```python
from build123d import *

# Parameters (mm, degrees)
SKETCH_1_W             = 67
SKETCH_1_H             = 62
EXTRUDE_1_DEPTH        = 10
SKETCH_3_W             = 14
SKETCH_3_H             = 20
EXTRUDE_2_DEPTH        = 12.5
SKETCH_4_W             = 10
SKETCH_4_H             = 65
EXTRUDE_3_DEPTH        = 67
SKETCH_5_W             = 67
SKETCH_5_H             = 44
EXTRUDE_4_DEPTH        = 8
EXTRUDE_5_DEPTH        = 20
CUT_EXTRUDE_START      = -6
CUT_EXTRUDE_1_DEPTH    = 8
EXTRUDE_6_DEPTH        = 6
SKETCH_9_R             = 3
CUT_EXTRUDE_2_DEPTH    = 23
SKETCH_10_W            = 24
SKETCH_10_H            = 23.8
EXTRUDE_7_DEPTH        = 8
SKETCH_12_W            = 14
SKETCH_12_H            = 20
EXTRUDE_8_DEPTH        = 11.5
SKETCH_13_R            = 0.95
CUT_EXTRUDE_4_DEPTH    = 8
SKETCH_14_W            = 8
SKETCH_14_H            = 6
EXTRUDE_9_DEPTH        = 11.8
SKETCH_15_R            = 0.95
CUT_EXTRUDE_5_DEPTH    = 11.8
SKETCH_16_W            = 3
SKETCH_16_H            = 6
EXTRUDE_10_DEPTH       = 12
FILLET_1_RADIUS        = 3
FILLET_1_LENGTH        = 3
SKETCH_17_R            = 1.75
CUT_EXTRUDE_6_DEPTH    = 7
SKETCH_18_R            = 3
EXTRUDE_11_DEPTH       = 36.5
FILLET_2_R             = 3
FILLET_2_OF_MIRROR_1_R = 3
SKETCH_20_R            = 1.75
CUT_EXTRUDE_7_DEPTH    = 35
SKETCH_21_W            = 15
SKETCH_21_H            = 55
CUT_EXTRUDE_8_DEPTH    = 35
SKETCH_24_R            = 1.75
CUT_EXTRUDE_11_DEPTH   = 18
SKETCH_25_R            = 1.5
CUT_EXTRUDE_12_DEPTH   = 10
FILLET_3_R             = 4
SKETCH_26_W            = 10.3
SKETCH_26_H            = 3.8
EXTRUDE_12_DEPTH       = 1
SKETCH_27_R            = 1.4
CUT_EXTRUDE_13_DEPTH   = 4


with BuildPart() as part:
    # 草图1 → 凸台-拉伸1 (new body)
    with BuildSketch(Plane(origin=(0, 0, 0), x_dir=(1, 0, 0), z_dir=(0, 1, 0))):
        Rectangle(SKETCH_1_W, SKETCH_1_H)
    extrude(amount=EXTRUDE_1_DEPTH)

    # 草图3 → 凸台-拉伸2 (add)
    with BuildSketch(Plane(origin=(0, 10, 0), x_dir=(1, 0, 0), z_dir=(0, 1, 0))):
        with Locations((-26.5, 26)):
            Rectangle(SKETCH_3_W, SKETCH_3_H)
    extrude(amount=EXTRUDE_2_DEPTH)

    # 草图4 → 凸台-拉伸3 (add)
    with BuildSketch(Plane.ZY.offset(33.5)):
        with Locations((-11, 42.5)):
            Rectangle(SKETCH_4_W, SKETCH_4_H)
    extrude(amount=-EXTRUDE_3_DEPTH)

    # 草图5 → 凸台-拉伸4 (add)
    with BuildSketch(Plane(origin=(0, 75, 0), x_dir=(1, 0, 0), z_dir=(0, 1, 0))):
        with Locations((0, -6)):
            Rectangle(SKETCH_5_W, SKETCH_5_H)
    extrude(amount=-EXTRUDE_4_DEPTH)

    # 草图6 → 凸台-拉伸5 (add)
    with BuildSketch(Plane(origin=(33.5, 0, 0), x_dir=(0, 0, -1), z_dir=(1, 0, 0))):
        with BuildLine():
            Line((-28, 60), (-28, 67))
            Line((-28, 67), (-8, 67))
            Line((-8, 67), (-8, 60))
            ThreePointArc((-8, 60), (-18, 50), (-28, 60))
        make_face()
    extrude_5 = extrude(amount=-EXTRUDE_5_DEPTH)

    # 草图7 → 切除-拉伸1 (cut)
    with BuildSketch(Plane(origin=(33.5, 0, 0), x_dir=(0, 0, -1), z_dir=(1, 0, 0)).offset(CUT_EXTRUDE_START)):
        with BuildLine():
            Line((-28, 60), (-28, 70.000230089))
            Line((-28, 70.000230089), (-8, 70.000230089))
            Line((-8, 70.000230089), (-8, 60))
            ThreePointArc((-8, 60), (-18, 50), (-28, 60))
        make_face()
    cut_extrude_1 = extrude(amount=-CUT_EXTRUDE_1_DEPTH, mode=Mode.SUBTRACT)

    # 草图8 → 凸台-拉伸6 (add)
    with BuildSketch(Plane(origin=(0, 75, 0), x_dir=(1, 0, 0), z_dir=(0, 1, 0))):
        Polygon((0, -68), (13, -68), (33.5, -28), (0, -28), align=None)
    extrude_6 = extrude(amount=-EXTRUDE_6_DEPTH)

    # 草图9 → 切除-拉伸2 (cut)
    with BuildSketch(Plane(origin=(33.5, 0, 0), x_dir=(0, 0, -1), z_dir=(1, 0, 0))):
        with Locations((-18, 60)):
            Circle(SKETCH_9_R)
    cut_extrude_2 = extrude(amount=-CUT_EXTRUDE_2_DEPTH, mode=Mode.SUBTRACT)

    # 草图10 → 凸台-拉伸7 (add)
    with BuildSketch(Plane(origin=(37.896299963, 0, 19.421853731), x_dir=(0.4560907909103985, 0, -0.8899332505568759), z_dir=(0.8899332505568758, 0, 0.45609079091039845))):
        Polygon((-44, 75), (-15, 75), (-15, 40.2), (-43, 40.2), (-49, 40.2), (-49, 75), align=None)
        with Locations((-32, 57.1)):
            Rectangle(SKETCH_10_W, SKETCH_10_H, mode=Mode.SUBTRACT)
    extrude_7 = extrude(amount=-EXTRUDE_7_DEPTH)

    # 草图12 → 凸台-拉伸8 (add)
    with BuildSketch(Plane(origin=(0, 75, 0), x_dir=(1, 0, 0), z_dir=(0, 1, 0))):
        with Locations((-26.5, 26)):
            Rectangle(SKETCH_12_W, SKETCH_12_H)
    extrude(amount=-EXTRUDE_8_DEPTH)

    # 草图13 → 切除-拉伸4 (cut)
    with BuildSketch(Plane(origin=(30.776833958, 0, 15.773127404), x_dir=(-0.4560907909103988, 0, 0.8899332505568758), z_dir=(-0.8899332505568757, 0, -0.4560907909103987))):
        with Locations((38.5, 70.95)):
            Circle(SKETCH_13_R)
        with Locations((26.5, 70.95)):
            Circle(SKETCH_13_R)
        with Locations((26.5, 43.25)):
            Circle(SKETCH_13_R)
        with Locations((38.5, 43.25)):
            Circle(SKETCH_13_R)
    cut_extrude_4 = extrude(amount=-CUT_EXTRUDE_4_DEPTH, mode=Mode.SUBTRACT)

    # 草图14 → 凸台-拉伸9 (add)
    with BuildSketch(Plane(origin=(0, 75, 0), x_dir=(1, 0, 0), z_dir=(0, 1, 0))):
        with Locations((7.7, -5)):
            Rectangle(SKETCH_14_W, SKETCH_14_H)
        with Locations((7.7, -34.8)):
            Rectangle(SKETCH_14_W, SKETCH_14_H)
    extrude(amount=EXTRUDE_9_DEPTH)

    # 草图15 → 切除-拉伸5 (cut)
    with BuildSketch(Plane.ZY.offset(-3.7)):
        with Locations((33.75, 81.5)):
            Circle(SKETCH_15_R)
        with Locations((6.05, 81.5)):
            Circle(SKETCH_15_R)
    extrude(amount=-CUT_EXTRUDE_5_DEPTH, mode=Mode.SUBTRACT)

    # 草图16 → 凸台-拉伸10 (add)
    with BuildSketch(Plane(origin=(0, 75, 0), x_dir=(1, 0, 0), z_dir=(0, 1, 0))):
        with Locations((0, -63)):
            Rectangle(SKETCH_16_W, SKETCH_16_H)
    extrude(amount=EXTRUDE_10_DEPTH)

    # 圆角1: full round fillet: the end face becomes a half cylinder, R = half its width
    fillet_1_face = Plane((0, 87, 63), x_dir=(1, 0, 0), z_dir=(0, 1, 0))  # on the end face: x along it, z out of the body
    fillet_1_slab = fillet_1_face.offset(-FILLET_1_RADIUS / 2) * Box(FILLET_1_LENGTH, 2 * FILLET_1_RADIUS, FILLET_1_RADIUS, mode=Mode.PRIVATE)  # the body's end, R deep
    fillet_1_round = Plane((0, 84, 63), x_dir=(0, 1, 0), z_dir=(1, 0, 0)) * Cylinder(FILLET_1_RADIUS, FILLET_1_LENGTH, mode=Mode.PRIVATE)  # its axis R under the face
    add(fillet_1_slab - fillet_1_round, mode=Mode.SUBTRACT)

    # 草图17 → 切除-拉伸6 (cut)
    with BuildSketch(Plane.ZY.offset(1.5)):
        with Locations((63, 84)):
            Circle(SKETCH_17_R)
    extrude(amount=-CUT_EXTRUDE_6_DEPTH, mode=Mode.SUBTRACT)

    # 草图18 → 凸台-拉伸11 (add)
    with BuildSketch(Plane(origin=(0, 75, 0), x_dir=(1, 0, 0), z_dir=(0, 1, 0))):
        with Locations(Location((10, 10, 0), (0, 0, 270))):
            Circle(SKETCH_18_R)
    extrude_11 = extrude(amount=EXTRUDE_11_DEPTH)

    # 圆角2
    fillet_2_edges = [part.edges().sort_by_distance(p)[0] for p in [
        (10, 75, -13),
    ]]
    fillet(fillet_2_edges, radius=FILLET_2_R - 0.0001)  # a hair under: the kernel refuses the full size

    # 镜向1: 凸台-拉伸5, 切除-拉伸1, 凸台-拉伸6, 切除-拉伸2, 凸台-拉伸7, 切除-拉伸4, 凸台-拉伸11 across plane
    add(extrude_5.mirror(Plane(origin=(0, 0, 0), x_dir=(0, 0, 1), z_dir=(1, 0, 0))))
    add(cut_extrude_1.mirror(Plane(origin=(0, 0, 0), x_dir=(0, 0, 1), z_dir=(1, 0, 0))), mode=Mode.SUBTRACT)
    add(extrude_6.mirror(Plane(origin=(0, 0, 0), x_dir=(0, 0, 1), z_dir=(1, 0, 0))))
    add(cut_extrude_2.mirror(Plane(origin=(0, 0, 0), x_dir=(0, 0, 1), z_dir=(1, 0, 0))), mode=Mode.SUBTRACT)
    add(extrude_7.mirror(Plane(origin=(0, 0, 0), x_dir=(0, 0, 1), z_dir=(1, 0, 0))))
    add(cut_extrude_4.mirror(Plane(origin=(0, 0, 0), x_dir=(0, 0, 1), z_dir=(1, 0, 0))), mode=Mode.SUBTRACT)
    add(extrude_11.mirror(Plane(origin=(0, 0, 0), x_dir=(0, 0, 1), z_dir=(1, 0, 0))))

    # 圆角2 of 镜向1
    fillet_2_of_mirror_1_edges = [part.edges().sort_by_distance(p)[0] for p in [
        (-10, 75, -13),
    ]]
    fillet(fillet_2_of_mirror_1_edges, radius=FILLET_2_OF_MIRROR_1_R - 0.0001)  # a hair under: the kernel refuses the full size

    # 草图20 → 切除-拉伸7 (cut)
    with BuildSketch(Plane.ZY.offset(33.5)):
        with Locations((-31, 67)):
            Circle(SKETCH_20_R)
        with Locations((-21, 67)):
            Circle(SKETCH_20_R)
        with Locations((-31, 19)):
            Circle(SKETCH_20_R)
        with Locations((-21, 19)):
            Circle(SKETCH_20_R)
    extrude(amount=-CUT_EXTRUDE_7_DEPTH, mode=Mode.SUBTRACT)

    # 草图21 → 切除-拉伸8 (cut)
    with BuildSketch(Plane(origin=(0, 0, -16), x_dir=(-1, 0, 0), z_dir=(0, 0, -1))):
        with Locations((0, 37.5)):
            Rectangle(SKETCH_21_W, SKETCH_21_H)
    extrude(amount=-CUT_EXTRUDE_8_DEPTH, mode=Mode.SUBTRACT)

    # 草图24 → 切除-拉伸11 (cut)
    with BuildSketch(Plane(origin=(0, 10, 0), x_dir=(1, 0, 0), z_dir=(0, 1, 0))):
        with Locations(Location((-10, -21, 0), (0, 0, 270))):
            Circle(SKETCH_24_R)
        with Locations(Location((10, -21, 0), (0, 0, 270))):
            Circle(SKETCH_24_R)
        with Locations(Location((-10, -1, 0), (0, 0, 270))):
            Circle(SKETCH_24_R)
        with Locations(Location((10, -1, 0), (0, 0, 270))):
            Circle(SKETCH_24_R)
    extrude(amount=-CUT_EXTRUDE_11_DEPTH, mode=Mode.SUBTRACT)

    # 草图25 → 切除-拉伸12 (cut)
    with BuildSketch(Plane(origin=(0, 111.5, 0), x_dir=(1, 0, 0), z_dir=(0, 1, 0))):
        with Locations(Location((10, 10, 0), (0, 0, 270))):
            Circle(SKETCH_25_R)
        with Locations(Location((-10, 10, 0), (0, 0, 270))):
            Circle(SKETCH_25_R)
    extrude(amount=-CUT_EXTRUDE_12_DEPTH, mode=Mode.SUBTRACT)

    # 圆角3
    fillet_3_edges = [part.edges().sort_by_distance(p)[0] for p in [
        (-1.5, 75, 63),
        (1.5, 75, 63),
    ]]
    fillet(fillet_3_edges, radius=FILLET_3_R)

    # 草图26 → 凸台-拉伸12 (add)
    with BuildSketch(Plane.XZ.offset(-69)):
        with Locations((0.05, 61.98)):
            Rectangle(SKETCH_26_W, SKETCH_26_H)
    extrude(amount=EXTRUDE_12_DEPTH)

    # 草图27 → 切除-拉伸13 (cut)
    with BuildSketch(Plane.XZ.offset(-68)):
        with Locations(Location((0.05, 62, 0), (0, 0, 270))):
            Circle(SKETCH_27_R)
    extrude(amount=-CUT_EXTRUDE_13_DEPTH, mode=Mode.SUBTRACT)


solid = part.part
```
Verification items for the finished model (mm, model axes). A direction names the side the tool comes from. Give positions to 0.01 mm unless a question says otherwise; leave off trailing zeros. Order: outer loops, then holes, each group sorted by start corner. A loop starts at its lowest first (then second) coordinate and runs counter-clockwise, first axis right, second up. Notation, with made-up numbers: (-21, -14.5) -> (-5, -14.5) arc R14 cw to (-5, -5.5) -> close; hole circle Ø5 at (27.5, 75.25). An arc over 180 degrees is marked (long way). One line per item, written item: value.
(1) Gauge pin test, flat ends, axial feed: pin 1 (5 mm diameter, centred on y = 78.5, z = 5.5, fed in from +X); pin 2 (17 mm diameter, centred on x = 1, y = 25.5, fed in from +Z); pin 3 (1.1 mm diameter, centred on y = 68.5, z = 63, fed in from -X); pin 4 (2 mm diameter, centred on x = -21.5, z = -5, fed in from -Y). Record the tip position at first contact, or that the pin passes through.
Final values:
pin 1: x = 11.7
pin 2: z = -6
pin 3: x = -15.84
pin 4: y = 0
(2) Scan lines: line 1 along X through (y, z) = (6, 21); line 2 along Y through (x, z) = (6.75, 33.75); line 3 along Y through (x, z) = (30.7, 18). Record each from-to range of solid material in increasing order. Write a range as [from, to].
Final values:
line 1: [-33.5, -11.75], [-8.25, 8.25], [11.75, 33.5]
line 2: [69, 80.55], [82.45, 86.8]
line 3: [0, 10], [50, 57], [63, 75]
(3) Draft check along Y on faces 1 (the face through (20, 45.2, 46)), 2 (the face through (-16.527, 42.407, 52.224)), 3 (the face through (11.7, 81, 5)). Enter one of: pulls with the +Y half, pulls with the -Y half, needs draft (parallel to the pull), parting line crosses it, or undercut.
Final values:
face 1: undercut
face 2: undercut
face 3: needs draft
(4) Sectioned sample at C-C on z = 12. Record the cut outline in (x, y), then the cut area to 3 significant figures.
Final values:
outline: (-33.5, 0) -> (33.5, 0) -> (33.5, 10) -> (-33.5, 10) -> close; (-33.5, 52) -> (-27.5, 52) -> (-27.5, 70) -> (-19.5, 70) -> (-19.5, 52) -> (-13.5, 52) -> (-13.5, 67) -> (13.5, 67) -> (13.5, 52) -> (19.5, 52) -> (19.5, 70) -> (27.5, 70) -> (27.5, 52) -> (33.5, 52) -> (33.5, 75) -> (-33.5, 75) -> close
area: 1,520 mm^2
(5) Tool access check on faces 4 (the face through (25.26, 56.93, 35.42)), 5 (the face through (14.32, 56.93, 56.78)), 6 (the face through (-10.9, 106.6, -11.2)). Record the directions out of +Z, -Z, +X, -X, +Y, -Y that give a thin tool (end or side, any length) a straight path to the whole face; none if there is none.
Final values:
face 4: +Z
face 5: +X
face 6: +Y
(6) Sectioned sample at A-A on x = 0.05. Record the cut outline in (y, z).
Final values:
outline: (0, -31) -> (10, -31) -> (10, 31) -> (0, 31) -> close; (65, -16) -> (75, -16) -> (75, 60) -> (84, 60) arc R3 ccw to (84, 66) -> (75, 66) -> (75, 68) -> (69, 68) -> (69, 63.88) -> (68, 63.88) -> (68, 63.4) -> (72, 63.4) -> (72, 60.6) -> (68, 60.6) -> (68, 60.08) -> (69, 60.08) -> (69, 28) -> (67, 28) -> (67, -6) -> (65, -6) -> close; hole circle Ø3.5 at (84, 63)
(7) Sectioned sample at B-B on y = 19. Record the cut outline in (x, z).
Final values:
outline: (-33.5, -36) -> (-19.5, -36) -> (-19.5, -32.75) -> (-33.5, -32.75) -> close; (-33.5, -29.25) -> (-19.5, -29.25) -> (-19.5, -22.75) -> (-33.5, -22.75) -> close; (-33.5, -19.25) -> (-19.5, -19.25) -> (-19.5, -16) -> (-7.5, -16) -> (-7.5, -6) -> (-33.5, -6) -> close; (7.5, -16) -> (33.5, -16) -> (33.5, -6) -> (7.5, -6) -> close
